Here's the drawing with two shaded views (mm, measured from the low corner). I have some questions. Round coordinates to 2 decimals unless told otherwise and drop trailing zeros. Loops run counter-clockwise (first coordinate to the right, second up) from the corner with the lowest first, then second, coordinate; pieces in that order, holes last. Notation, with made-up numbers: (6.25, 58) -> (15.25, 58) arc R21 cw to (15.25, 85) -> close; hole circle Ø10 at (3, -29). An arc over 180 degrees is marked (long way). Use a Markdown table: item, result.
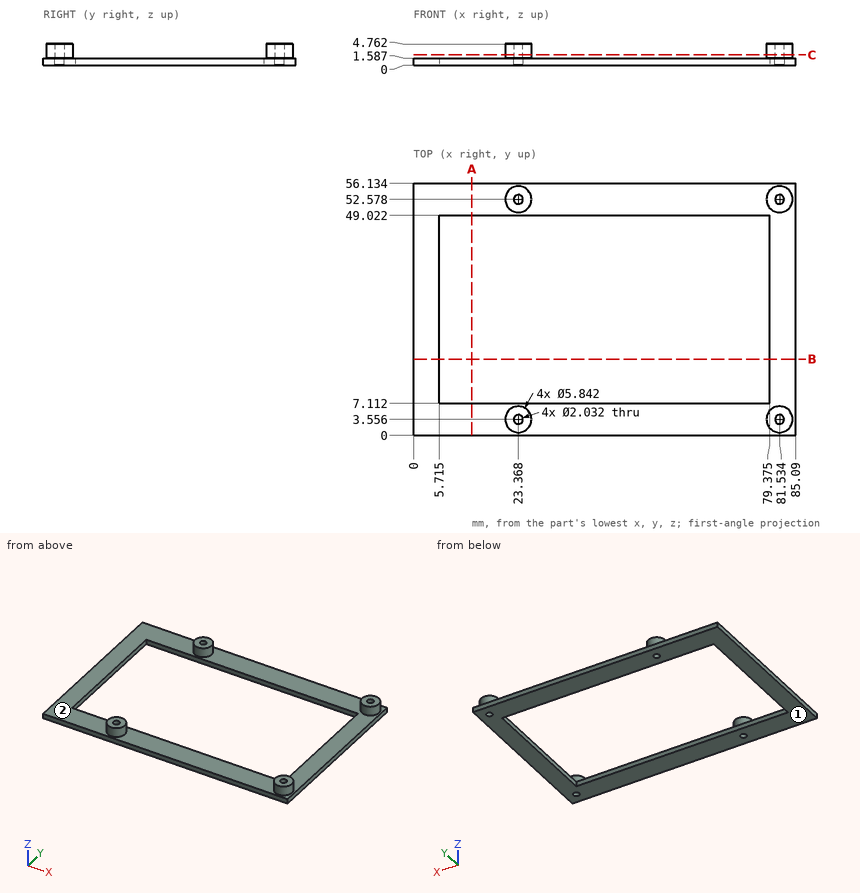
1. I want a section at B-B (y = 17). Please give me the cut outline in (x, z) (1 decimal).
Answer sheet:
| item | result |
|---|---|
| outline | (0, 0) -> (5.7, 0) -> (5.7, 1.6) -> (0, 1.6) -> close; (79.4, 0) -> (85.1, 0) -> (85.1, 1.6) -> (79.4, 1.6) -> close |
2. I need wall thicknesses on line 1 (Y direction, x = 62, z = 0.9) (1 decimal); line 2 (X direction, y = 31.5, z = 0.6) (1 decimal); line 3 (X direction, y = 53, z = 2.35) (1 decimal). Which ranges of each line are inside material? Lowest first, please.
Answer sheet:
| item | result |
|---|---|
| line 1 | y = 0 to 7.1, 49 to 56.1 |
| line 2 | x = 0 to 5.7, 79.4 to 85.1 |
| line 3 | x = 20.5 to 22.4, 24.3 to 26.3, 78.6 to 80.6, 82.5 to 84.4 |
3. I want a section at A-A (x = 13). Please give me the cut outline in (y, z) (1 decimal).
Answer sheet:
| item | result |
|---|---|
| outline | (0, 0) -> (7.1, 0) -> (7.1, 1.6) -> (0, 1.6) -> close; (49, 0) -> (56.1, 0) -> (56.1, 1.6) -> (49, 1.6) -> close |
4. If we mould it in two halves opening along X, with no side actions, what happens to the marked faces 1 and 2? For each: +X half, -X half, draft (parallel to the pull), parting line (faces both ways), or undercut.
Answer sheet:
| item | result |
|---|---|
| face 1 | draft |
| face 2 | undercut |
5. I want a section at C-C (z = 2.35). State how many separate pieces and enclosed holes the cut face has.
Answer sheet:
| item | result |
|---|---|
| separate pieces | 4 |
| enclosed holes | 4 |
6. Will this pin go through, and if not, where does the flat tip stop? pin 1 Ø2 at (y, z) = (8.5, 3.5) entering from +X.
Answer sheet:
| item | result |
|---|---|
| pin 1 | passes through |
